Verification items for the finished model (mm, model axes). Face numbers are marked on the shaded views. A direction names the side the tool comes from. Give positions to 0.01 mm unless a question says otherwise; leave off trailing zeros. Order: outer loops, then holes, each group sorted by start corner. A loop starts at its lowest first (then second) coordinate and runs counter-clockwise, first axis right, second up. Notation, with made-up numbers: M 13.5,-2 L 27.5,-2 A12 cw 27.5,10 Z; hole C -4.5,60 d2. An arc over 180 degrees is marked long. Answer as a JSON object with one key per item and string values.
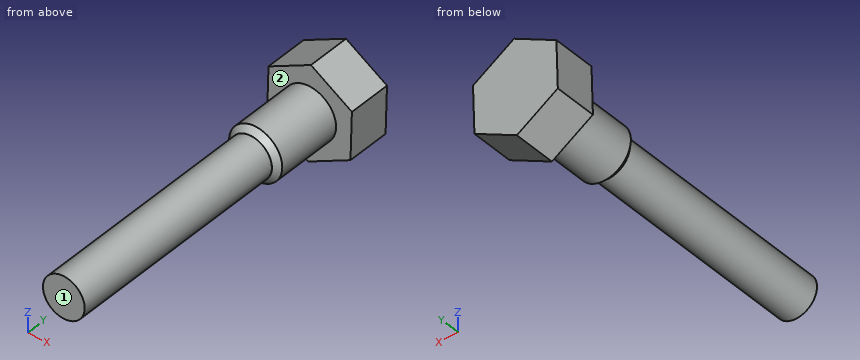
```python
from build123d import *

# Parameters (mm, degrees)
F1_DEPTH = 38.1
F2_R     = 23.922901
F3_DEPTH = 63.5
F4_SIZE  = 5.08
F5_R     = 18.798033
F6_DEPTH = 203.2


with BuildPart() as f1:
    # F0 (on Front) → F1 (new body)
    with BuildSketch(Plane.XZ):
        Polygon((1.283812, 43.336898), (-36.888948, 22.780262), (-38.17276, -20.556635), (-1.283812, -43.336898), (36.888948, -22.780262), (38.17276, 20.556635), align=None)
    extrude(amount=F1_DEPTH)

    # F2 (on face) → F3 (join)
    with BuildSketch(Plane.XZ.offset(38.1)):
        Circle(F2_R)
    extrude(amount=F3_DEPTH)

    # F4
    f4_edges = [f1.edges().sort_by_distance(p)[0] for p in [
        (-23.922901, -101.6, 0),
    ]]
    chamfer(f4_edges, length=F4_SIZE)

    # F5 (on face) → F6 (join)
    with BuildSketch(Plane.XZ.offset(101.6)):
        Circle(F5_R)
    extrude(amount=F6_DEPTH)


solid = f1.part
```
Q1. Gauge pin test, flat ends, axial feed: pin 1 Ø10 at (y, z) = (-145.5, -12) entering from +X; pin 2 Ø5 at (x, z) = (22, -10.5) entering from -Y; pin 3 Ø10 at (y, z) = (-175, 17) entering from +X; pin 4 Ø8 at (x, y) = (-26, -102.5) entering from -Z. Record the tip position at first contact, or that the pin passes through.
Resolved:
{"pin 1": "stops at x = 17.45", "pin 2": "stops at y = -98.57", "pin 3": "stops at x = 14.47", "pin 4": "passes through"}
Q2. Section check B-B on y = -67. Record the cut outline in (x, z), then the cut area to 3 significant figures.
Resolved:
{"outline": "C 0,0 d47.85", "area": "1,800 mm²"}
Q3. Section check C-C on y = -143. Record the cut outline in (x, z).
Resolved:
{"outline": "C 0,0 d37.6"}
Q4. Section check D-D on z = 31. Record the cut outline in (x, y), then the cut area to 3 significant figures.
Resolved:
{"outline": "M -21.63,-38.1 L 21.26,-38.1 L 21.26,0 L -21.63,0 Z", "area": "1,630 mm²"}
Q5. Tool access check on the marked faces 1 and 2. Record the directions out of +Z, -Z, +X, -X, +Y, -Y that give a thin tool (end or side, any length) a straight path to the whole face; none if there is none.
Resolved:
{"face 1": "+Z, -Z, +X, -X, -Y", "face 2": "-Y"}
Q6. Section check A-A on z = 0. Record the cut outline in (x, y).
Resolved:
{"outline": "M -37.56,-38.1 L -23.92,-38.1 L -23.92,-96.52 L -18.84,-101.6 L -18.8,-101.6 L -18.8,-304.8 L 18.8,-304.8 L 18.8,-101.6 L 18.84,-101.6 L 23.92,-96.52 L 23.92,-38.1 L 37.56,-38.1 L 37.56,0 L -37.56,0 Z"}
Q7. Material ranges on L1, parallel to Y at x = 28.5, z = -25.5; L2, parallel to X at y = -260, z = 0.5; L3, parallel to Y at x = -5, z = 23, recorded low to high.
Resolved:
{"L1": "y = -38.1 to 0", "L2": "x = -18.79 to 18.79", "L3": "y = -96.91 to 0"}
